Work out the finished part from the listing and answer in its coordinate system (mm). A direction names the side the tool comes from. Round coordinates to 2 decimals unless told otherwise and drop trailing zeros. Loops run counter-clockwise (first coordinate to the right, second up) from the corner with the lowest first, then second, coordinate; pieces in that order, holes last. Notation, with made-up numbers: (86, 20.25) -> (108, 20.25) arc R32 ccw to (108, 52.25) -> close; hole circle Ø9 at (44.5, 75). An arc over 180 degrees is marked (long way). Use one line per item in the form item = value.
```python
from build123d import *

# Parameters (mm, degrees)
SKETCH1_R           = 5
BOSS_EXTRUDE1_DEPTH = 104
BOSS_EXTRUDE2_DEPTH = 100
BOSS_EXTRUDE3_START = -104
BOSS_EXTRUDE3_DEPTH = 40


with BuildPart() as part:
    # Sketch1 → Boss-Extrude1 (new body)
    with BuildSketch(Plane(origin=(0, 0, 0), x_dir=(1, 0, 0), z_dir=(0, 1, 0))):
        Circle(SKETCH1_R)
    extrude(amount=BOSS_EXTRUDE1_DEPTH)

    # Sketch2 → Boss-Extrude2 (add)
    with BuildSketch(Plane(origin=(0, 104, 0), x_dir=(1, 0, 0), z_dir=(0, 1, 0))):
        with BuildLine():
            Line((-2, 4.582576), (-2, -4.582576))
            ThreePointArc((-2, -4.582576), (-5, 0), (-2, 4.582576))
        make_face()
        with BuildLine():
            Line((2, 4.582576), (2, -4.582576))
            ThreePointArc((2, -4.582576), (5, 0), (2, 4.582576))
        make_face()
    extrude(amount=BOSS_EXTRUDE2_DEPTH)

    # Sketch2<2> → Boss-Extrude3 (add)
    with BuildSketch(Plane(origin=(0, 104, 0), x_dir=(1, 0, 0), z_dir=(0, 1, 0)).offset(BOSS_EXTRUDE3_START)):
        with BuildLine():
            Line((-2, 4.582576), (-2, -4.582576))
            ThreePointArc((-2, -4.582576), (-5, 0), (-2, 4.582576))
        make_face()
        with BuildLine():
            Line((2, 4.582576), (2, -4.582576))
            ThreePointArc((2, -4.582576), (5, 0), (2, 4.582576))
        make_face()
    extrude(amount=-BOSS_EXTRUDE3_DEPTH)


solid = part.part
```
(1) For faces 1 (the flat face through (-2, 153, 0)), 2 (the flat face through (0, 0, 0)), determine the directions among +Z, -Z, +X, -X, +Y, -Y from which every point of the face is accessible in a straight line to the end or side of a thin tool.
Completed:
face_1 = +Z, -Z, +Y
face_2 = +Z, -Z, -Y
(2) Find section A-A, the plane z = 3. Write down the section's boundary in (x, y), then the cut area to 3 significant figures.
Completed:
outline = (-4, -40) -> (-2, -40) -> (-2, 0) -> (2, 0) -> (2, -40) -> (4, -40) -> (4, 204) -> (2, 204) -> (2, 104) -> (-2, 104) -> (-2, 204) -> (-4, 204) -> close
area = 1,390 mm2
(3) Find section D-D, the plane y = 31.5. Write down the section's boundary in (x, z).
Completed:
outline = circle Ø10 at (0, 0)
(4) Given P1, Ø1, axis at y = 28.5, z = 2, coming from the -X side; P2, Ø2, axis at x = 0.5, z = -1, coming from the +Y side; P3, Ø5, axis at x = 0, z = -1, coming from the +Y side; P4, Ø2.5, axis at y = 131, z = 2, coming from the +X side, each flat-ended and moving along its own axis, determine where each tip first touches the part or whether it passes through.
Completed:
P1 = -4.77
P2 = 104
P3 = 204
P4 = 4.94
(5) Consider L1, parallel to X at y = 111.5, z = 0.5; L2, parallel to Y at x = -0.75, z = -0.5; L3, parallel to X at y = 53, z = -2. Determine where each line is inside the solid, lowest interval first.
Completed:
L1 = -4.97 to -2, 2 to 4.97
L2 = 0 to 104
L3 = -4.58 to 4.58
(6) Find section C-C, the plane x = -3.5. Write down the section's boundary in (y, z).
Completed:
outline = (-40, -3.57) -> (204, -3.57) -> (204, 3.57) -> (-40, 3.57) -> close
(7) Find section B-B, the plane y = 124.5. Write down the section's boundary in (x, z).
Completed:
outline = (-2, -4.58) -> (-2, 4.58) arc R5 ccw to start; (2, -4.58) arc R5 ccw to (2, 4.58) -> close
